Model file for the job. Use its own axes, mm. Give positions to 0.01 mm unless a question says otherwise; leave off trailing zeros. Loops run counter-clockwise (first coordinate to the right, second up) from the corner with the lowest first, then second, coordinate; pieces in that order, holes last. Notation, with made-up numbers: (34.5, 16.25) - (52.5, 16.25) arc R38 cw to (52.5, 54.25) - close; hole circle Ø9 at (49.5, -40). An arc over 180 degrees is marked (long way). Answer as CSV lines item,"result". Start each with the question number.
Item 1: Drill centre lines: L1, parallel to X at y = 24.75, z = 1.2; L2, parallel to X at y = 25, z = 1.6; L3, parallel to Y at x = 105, z = 1.45. Where is each one in solid material? Low to high. Write a range as from..to.
Item 2: Saw through at A-A on z = 0.6. Give the cut face in (x, y), plus the area to 3 significant figures.
Item 3: Pin check, flat tips, straight feed: pin 1 (4 mm diameter, centred on x = 31.32, y = 25.1, fed in from +Z); pin 2 (1 mm diameter, centred on y = 24, z = 1, fed in from -X); pin 3 (1.8 mm diameter, centred on x = 111.31, y = 26.09, fed in from -Z). Stop position of each tip, or through.
Item 4: Saw through at B-B on x = 99. Give the cut face in (y, z), plus the area to 3 significant figures.
Item 5: Saw through at C-C on x = 77. Give the cut face in (y, z), plus the area to 3 significant figures.
from build123d import *

# Parameters (mm, degrees)
MODEL_R             = 1.5
BOSS_EXTRUDE1_DEPTH = 3


with BuildPart() as part:
    # Model → Boss-Extrude1 (new body)
    with BuildSketch(Plane.XY):
        with BuildLine():
            Line((49.968489673, 21.049962128), (105.618768597, 21.289392046))
            ThreePointArc((105.618768597, 21.289392046), (107.285112204, 21.118249382), (108.87926509, 20.60379102))
            ThreePointArc((108.87926509, 20.60379102), (117.192196904, 26.162159278), (108.74462654, 31.51368691))
            ThreePointArc((108.74462654, 31.51368691), (107.163632348, 30.960034557), (105.502006567, 30.747729758))
            Line((105.502006567, 30.747729758), (31.227056592, 29.101105192))
            ThreePointArc((31.227056592, 29.101105192), (28.246037105, 27.617586299), (27.362873685, 24.407083556))
            ThreePointArc((27.362873685, 24.407083556), (28.356080114, 22.511229951), (30.031202973, 21.179057549))
            ThreePointArc((30.031202973, 21.179057549), (30.946620491, 21.021963969), (31.874075806, 20.972021358))
            Line((31.874075806, 20.972021358), (49.968489673, 21.049962128))
        make_face()
        with Locations((31.31571206, 25.102087789)):
            Circle(MODEL_R, mode=Mode.SUBTRACT)
        with Locations((111.309575273, 26.089603674)):
            Circle(MODEL_R, mode=Mode.SUBTRACT)
    extrude(amount=BOSS_EXTRUDE1_DEPTH)


solid = part.part
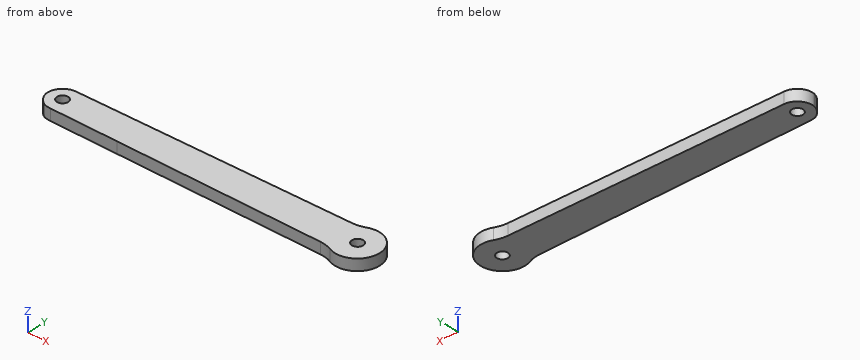
Responses:
1,L1,"27.33..29.86, 32.77..110.63, 111.98..117.04"
1,L2,"27.32..29.82, 32.81..110.28, 112.34..117.09"
1,L3,"21.29..30.74"
2,outline,"(27.36, 24.41) arc R5.18 ccw to (30.03, 21.18) arc R8 ccw to (31.87, 20.97) - (49.97, 21.05) - (105.62, 21.29) arc R8 cw to (108.88, 20.6) arc R5.97 ccw (long way) to (108.74, 31.51) arc R8 cw to (105.5, 30.75) - (31.23, 29.1) arc R4.08 ccw to start; hole circle Ø3 at (31.32, 25.1); hole circle Ø3 at (111.31, 26.09)"
2,area,"780 mm2"
3,pin 1,"z = 3"
3,pin 2,"x = 27.35"
3,pin 3,"through"
4,outline,"(21.26, 0) - (30.6, 0) - (30.6, 3) - (21.26, 3) - close"
4,area,"28.0 mm2"
5,outline,"(21.17, 0) - (30.12, 0) - (30.12, 3) - (21.17, 3) - close"
5,area,"26.8 mm2"
